Design review of the part built by this model. Coordinates are the model's own, in mm. A direction names the side the tool comes from. Coordinates: 2 decimals unless noted, no trailing zeros. Write each loop counter-clockwise with the first axis right and the second up, starting at its lowest first coordinate (ties: lowest second). Pieces come first, ordered by that corner, then holes. Notation, with made-up numbers: (27.25, 38.25) - (71.25, 38.25) arc R23 ccw to (71.25, 72.25) - close; hole circle Ø10 at (73.5, 48). An arc over 180 degrees is marked (long way). Answer as a JSON object with one key per item and string values.
```python
from build123d import *

# Parameters (mm, degrees)
BOSS_EXTRUDE1_DEPTH      = 350
SKETCH7_R                = 10.999999996
CUT_EXTRUDE1_DEPTH       = 355.660400947
SKETCH8_R                = 1.499999996
CUT_EXTRUDE2_DEPTH       = 355.660400947
F_3_0_3_DIAMETER_HOLE1_D = 3


with BuildPart() as part:
    # Sketch1 → Boss-Extrude1 (new body)
    with BuildSketch(Plane.XY):
        Polygon((0, 0), (0, 30), (2, 30), (2, 2), (50, 2), (50, 0), align=None)
    extrude(amount=BOSS_EXTRUDE1_DEPTH)

    # Sketch7 → Cut-Extrude1 (cut, through all)
    with BuildSketch(Plane(origin=(0, 2, 0), x_dir=(1, 0, 0), z_dir=(0, 1, 0))):
        with Locations(Location((26, -175, 0), (0, 0, 90))):
            Circle(SKETCH7_R)
    extrude(amount=-CUT_EXTRUDE1_DEPTH, mode=Mode.SUBTRACT)

    # Sketch8 → Cut-Extrude2 (cut, through all)
    with BuildSketch(Plane(origin=(0, 2, 0), x_dir=(1, 0, 0), z_dir=(0, 1, 0))):
        with Locations(Location((41.5, -190.5, 0), (0, 0, 270))):
            Circle(SKETCH8_R)
        with Locations(Location((41.5, -159.5, 0), (0, 0, 270))):
            Circle(SKETCH8_R)
        with Locations(Location((10.5, -190.5, 0), (0, 0, 270))):
            Circle(SKETCH8_R)
        with Locations(Location((10.5, -159.5, 0), (0, 0, 270))):
            Circle(SKETCH8_R)
    extrude(amount=-CUT_EXTRUDE2_DEPTH, mode=Mode.SUBTRACT)

    # Ø3.0 (3) Diameter Hole1 (through all)
    with Locations(Plane(origin=(0, 182.32004832, 128.861996081), x_dir=(0, 0, -1), z_dir=(-1, 0, 0))):
        with Locations((105.861996081, 174.32004832), (105.861996081, 157.32004832), (120.861996081, 167.32004832)):
            Hole(F_3_0_3_DIAMETER_HOLE1_D / 2)


solid = part.part
```
(1) The part is to be moulded in two halves that separate along Z. For faces 3 (the face through (14, 0, 173)), 4 (the face through (26, 1, 186)), 5 (the face through (17.7, 1.7, 350)), 6 (the face through (17.7, 1.7, 0)), say which applies: pulls with the +Z half, pulls with the -Z half, needs draft (parallel to the pull), parting line crosses it, or undercut.
Solved:
{"face 3": "needs draft", "face 4": "undercut", "face 5": "pulls with the +Z half", "face 6": "pulls with the -Z half"}
(2) Take a section at A-A, the plane z = 175. Write out the cut boundary in (x, y), and give its area (3 significant figures).
Solved:
{"outline": "(0, 0) - (15, 0) - (15, 2) - (2, 2) - (2, 30) - (0, 30) - close; (37, 0) - (50, 0) - (50, 2) - (37, 2) - close", "area": "112 mm^2"}
(3) To check wall thickness, follow line 1 (X direction, y = 1.2, z = 159.5); line 2 (Y direction, x = 0.5, z = 23); line 3 (Y direction, x = 16.5, z = 330). State the ranges of each line that lie inside material, in increasing order. Write a range as from..to.
Solved:
{"line 1": "x = 0..9, 12..40, 43..50", "line 2": "y = 0..6.5, 9.5..23.5, 26.5..30", "line 3": "y = 0..2"}
(4) Take a section at B-B, the plane z = 118.5. Write out the cut boundary in (x, y).
Solved:
{"outline": "(0, 0) - (50, 0) - (50, 2) - (2, 2) - (2, 30) - (0, 30) - close"}
(5) For pin 1 (14.5 mm diameter, centred on x = 33, z = 199, fed in from +Y); pin 2 (4 mm diameter, centred on x = 41.5, z = 159.5, fed in from -Y); pin 3 (5 mm diameter, centred on y = 25, z = 23, fed in from +X); pin 4 (20 mm diameter, centred on x = 26, z = 175, fed in from +Y), all flat-tipped, find the tip position at first contact; note any pin that passes through.
Solved:
{"pin 1": "stops at y = 2", "pin 2": "stops at y = 0", "pin 3": "stops at x = 2", "pin 4": "passes through"}
(6) Take a section at C-C, the plane y = 20.5. Write out the cut boundary in (x, z).
Solved:
{"outline": "(0, 0) - (2, 0) - (2, 350) - (0, 350) - close"}
(7) Tool access review of faces 1 (the face through (15, 2, 173)), 2 (the face through (0, 15, 173)): name each direction out of +Z, -Z, +X, -X, +Y, -Y from which nothing blocks a thin tool from reaching the whole face with its end or side.
Solved:
{"face 1": "+Z, -Z, +X, +Y", "face 2": "+Z, -Z, -X, +Y, -Y"}
